Verification items for the finished model (mm, model axes). A direction names the side the tool comes from. Coordinates: 2 decimals unless noted, no trailing zeros. Write each loop counter-clockwise with the first axis right and the second up, starting at its lowest first coordinate (ties: lowest second). Pieces come first, ordered by that corner, then holes. Notation, with made-up numbers: (-2.75, 25.5) -> (10.25, 25.5) arc R7 cw to (10.25, 31.5) -> close; hole circle Ø8 at (72, -40). An arc over 180 degrees is marked (long way). Answer in a Markdown table with one row per item.
```python
from build123d import *

# Parameters (mm, degrees)
SZKIC1_W                    = 180
SZKIC1_H                    = 175
SZKIC1_R                    = 5
SZKIC1_R_2                  = 2.75
DODANIE_WYCI_GNI_CIE1_DEPTH = 3
SZKIC1_4_W                  = 180
SZKIC1_4_H                  = 175
SZKIC1_4_R                  = 5
DODANIE_WYCI_GNI_CIE2_DEPTH = 20
ZAOKR_GLENIE1_R             = 5


with BuildPart() as part:
    # Szkic1 → Dodanie-wyciągnięcie1 (new body)
    # profile 1 of 5: a face of its own
    with BuildSketch(Plane(origin=(0, 0, 0), x_dir=(1, 0, 0), z_dir=(0, 1, 0))):
        Rectangle(SZKIC1_W, SZKIC1_H)
        with Locations((70, -77.5)):
            Circle(SZKIC1_R, mode=Mode.SUBTRACT)
        with Locations((-70, -77.5)):
            Circle(SZKIC1_R, mode=Mode.SUBTRACT)
        with Locations((70, 77.5)):
            Circle(SZKIC1_R, mode=Mode.SUBTRACT)
        with Locations((-70, 77.5)):
            Circle(SZKIC1_R, mode=Mode.SUBTRACT)
    # profile 2 of 5: a face of its own
    with BuildSketch(Plane(origin=(0, 0, 0), x_dir=(1, 0, 0), z_dir=(0, 1, 0))):
        with Locations((-70, -77.5)):
            Circle(SZKIC1_R)
        with Locations(Location((-70, -77.5, 0), (0, 0, 270))):
            Circle(SZKIC1_R_2, mode=Mode.SUBTRACT)
    # profile 3 of 5: a face of its own
    with BuildSketch(Plane(origin=(0, 0, 0), x_dir=(1, 0, 0), z_dir=(0, 1, 0))):
        with Locations((-70, 77.5)):
            Circle(SZKIC1_R)
        with Locations(Location((-70, 77.5, 0), (0, 0, 270))):
            Circle(SZKIC1_R_2, mode=Mode.SUBTRACT)
    # profile 4 of 5: a face of its own
    with BuildSketch(Plane(origin=(0, 0, 0), x_dir=(1, 0, 0), z_dir=(0, 1, 0))):
        with Locations((70, 77.5)):
            Circle(SZKIC1_R)
        with Locations(Location((70, 77.5, 0), (0, 0, 270))):
            Circle(SZKIC1_R_2, mode=Mode.SUBTRACT)
    # profile 5 of 5: a face of its own
    with BuildSketch(Plane(origin=(0, 0, 0), x_dir=(1, 0, 0), z_dir=(0, 1, 0))):
        with Locations((70, -77.5)):
            Circle(SZKIC1_R)
        with Locations(Location((70, -77.5, 0), (0, 0, 270))):
            Circle(SZKIC1_R_2, mode=Mode.SUBTRACT)
    extrude(amount=DODANIE_WYCI_GNI_CIE1_DEPTH)

    # Szkic1<4> → Dodanie-wyciągnięcie2 (add)
    with BuildSketch(Plane(origin=(0, 0, 0), x_dir=(1, 0, 0), z_dir=(0, 1, 0))):
        Rectangle(SZKIC1_4_W, SZKIC1_4_H)
        with Locations(Location((70, -77.5, 0), (0, 0, 270))):
            Circle(SZKIC1_4_R, mode=Mode.SUBTRACT)
        with Locations(Location((-70, -77.5, 0), (0, 0, 270))):
            Circle(SZKIC1_4_R, mode=Mode.SUBTRACT)
        with Locations(Location((70, 77.5, 0), (0, 0, 270))):
            Circle(SZKIC1_4_R, mode=Mode.SUBTRACT)
        with Locations(Location((-70, 77.5, 0), (0, 0, 270))):
            Circle(SZKIC1_4_R, mode=Mode.SUBTRACT)
    extrude(amount=DODANIE_WYCI_GNI_CIE2_DEPTH)

    # Zaokrąglenie1
    zaokr_glenie1_edges = [part.edges().sort_by_distance(p)[0] for p in [
        (0, 20, 87.5),
    ]]
    fillet(zaokr_glenie1_edges, radius=ZAOKR_GLENIE1_R - 0.0001)  # a hair under: the kernel refuses the full size


solid = part.part
```
1. Sectioned sample at B-B, the plane x = -70. Count the separate pieces of the cut face and the enclosed holes in it, and give its area (3 significant figures).
Findings below:
| item | result |
|---|---|
| separate pieces | 3 |
| enclosed holes | 0 |
| area | 3,120 mm² |
2. Go/stop test with a flat-tipped pin: pin 1 (3 mm diameter, centred on x = 68.5, z = -77, fed in from +Y). Record where the tip stops, or that it passes through.
Findings below:
| item | result |
|---|---|
| pin 1 | stops at y = 3 |
3. Material ranges on probe 1 along Z at (x, y) = (-70, 11); probe 2 along X at (y, z) = (15.25, 77.5); probe 3 along X at (y, z) = (18, -76), recorded low to high. Write a range as from..to.
Findings below:
| item | result |
|---|---|
| probe 1 | z = -87.5..-82.5, -72.5..72.5, 82.5..87.5 |
| probe 2 | x = -90..-75, -65..65, 75..90 |
| probe 3 | x = -90..-74.77, -65.23..65.23, 74.77..90 |
4. Access from +Z, -Z, +X, -X, +Y, -Y to the whole of each face (thin tool, end or side, straight path). Record for faces 1 (the face through (-68.5, 11.38, 82.27)), 2 (the face through (-1, 20, -4)).
Findings below:
| item | result |
|---|---|
| face 1 | +Y |
| face 2 | +Z, -Z, +X, -X, +Y |
5. Release check for a two-part mould opening along X. For faces 3 (the face through (1.26, 18.57, 86)), 4 (the face through (90, 10, 1)), 5 (the face through (72, 3, 80)) record: released by +X, released by -X, zero draft, split by the parting line, or undercut.
Findings below:
| item | result |
|---|---|
| face 3 | zero draft |
| face 4 | released by +X |
| face 5 | undercut |
6. Sectioned sample at A-A, the plane z = -77.5. Record the cut outline in (x, y).
Findings below:
| item | result |
|---|---|
| outline | (-90, 0) -> (-72.75, 0) -> (-72.75, 3) -> (-75, 3) -> (-75, 20) -> (-90, 20) -> close; (-67.25, 0) -> (67.25, 0) -> (67.25, 3) -> (65, 3) -> (65, 20) -> (-65, 20) -> (-65, 3) -> (-67.25, 3) -> close; (72.75, 0) -> (90, 0) -> (90, 20) -> (75, 20) -> (75, 3) -> (72.75, 3) -> close |
